```python
from build123d import *

# Parameters (mm, degrees)
BOSS_EXTRUDE1_DEPTH      = 10
BOSS_EXTRUDE2_DEPTH      = 1
BOSS_EXTRUDE2_DEPTH_BACK = 11
BOSS_EXTRUDE3_DEPTH      = 5
BOSS_EXTRUDE3_DEPTH_BACK = 5
BOSS_EXTRUDE4_DEPTH      = 5
BOSS_EXTRUDE4_DEPTH_BACK = 5
SKETCH19_R               = 1
CUT_EXTRUDE3_DEPTH       = 10
SKETCH24_R               = 1
CUT_EXTRUDE4_DEPTH       = 10
REVOLVE2_ANGLE           = 90
CUT_REVOLVE4_ANGLE       = 80


with BuildPart() as part:
    # Sketch1 → Boss-Extrude1 (new body)
    with BuildSketch(Plane.XY):
        with BuildLine():
            Line((186.280110435, 212.216863761), (189.127439812, 0))
            Line((189.127439812, 0), (0, 0))
            Line((0, 0), (0, 125.576698411))
            add(Edge.make_bspline(
                [(0, 125.576698411), (10.557001905, 132.837635912), (17.098165485, 150.751131911), (30.538510921, 175.76338894), (49.352217031, 203.04075133), (76.867896029, 207.296992896), (91.097956951, 209.776295723)],
                knots=[0, 0, 0, 0, 0.275246051, 0.426571591, 0.655828837, 1, 1, 1, 1], degree=3))
            add(Edge.make_bspline(
                [(91.097956951, 209.776295723), (122.565116695, 215.374757588), (154.60100966, 210.515513687), (186.280110435, 212.216863761)],
                knots=[0, 0, 0, 0, 1, 1, 1, 1], degree=3))
        make_face()
    extrude(amount=BOSS_EXTRUDE1_DEPTH)

    # Sketch3 → Boss-Extrude2 (add, two sides)
    with BuildSketch(Plane.XY.offset(10)) as boss_extrude2_sk:
        with BuildLine():
            Line((40.691917073, 127.565231362), (173.80372619, 127.565231362))
            Line((173.80372619, 127.565231362), (173.80372619, 199.679337801))
            add(Edge.make_bspline(
                [(40.691917073, 127.565231362), (46.771290341, 134.933306827), (53.369134393, 161.704453989), (78.457507643, 191.212262771), (124.31750344, 201.038762955), (152.264868916, 199.362802741), (173.80372619, 199.679337801)],
                knots=[0, 0, 0, 0, 0.16561761, 0.500501685, 0.611599227, 1, 1, 1, 1], degree=3))
        make_face()
    extrude(amount=BOSS_EXTRUDE2_DEPTH)
    extrude(boss_extrude2_sk.sketch, amount=-BOSS_EXTRUDE2_DEPTH_BACK)

    # Sketch17 → Boss-Extrude3 (add, two sides)
    with BuildSketch(Plane(origin=(0, 40, 0), x_dir=(-1, 0, 0), z_dir=(0, -1, 0))) as boss_extrude3_sk:
        with BuildLine():
            Line((-188.57501815, 0), (-189.57501815, 0))
            ThreePointArc((-189.57501815, 0), (-192.762810227, -4.99036016), (-189.57501815, -9.98072032))
            Line((-189.57501815, -9.98072032), (-188.57501815, -9.98072032))
            Line((-188.57501815, -9.98072032), (-188.57501815, 0))
        make_face()
    extrude(amount=BOSS_EXTRUDE3_DEPTH)
    extrude(boss_extrude3_sk.sketch, amount=-BOSS_EXTRUDE3_DEPTH_BACK)

    # Sketch18 → Boss-Extrude4 (add, two sides)
    with BuildSketch(Plane(origin=(0, 160, 0), x_dir=(-1, 0, 0), z_dir=(0, -1, 0))) as boss_extrude4_sk:
        with BuildLine():
            Line((-186.972854644, -10), (-187.472854644, -10))
            ThreePointArc((-187.472854644, -10), (-190.720096746, -5), (-187.472854644, 0))
            Line((-187.472854644, 0), (-186.972854644, 0))
            Line((-186.972854644, 0), (-186.972854644, -10))
        make_face()
    extrude(amount=BOSS_EXTRUDE4_DEPTH)
    extrude(boss_extrude4_sk.sketch, amount=-BOSS_EXTRUDE4_DEPTH_BACK)

    # Sketch19 → Cut-Extrude3 (cut)
    with BuildSketch(Plane.XZ.offset(-155)):
        with Locations((188.57501815, 5)):
            Circle(SKETCH19_R)
    extrude(amount=-CUT_EXTRUDE3_DEPTH, mode=Mode.SUBTRACT)

    # Sketch24 → Cut-Extrude4 (cut)
    with BuildSketch(Plane.XZ.offset(-35)):
        with Locations((190.94512502, 4.99518008)):
            Circle(SKETCH24_R)
    extrude(amount=-CUT_EXTRUDE4_DEPTH, mode=Mode.SUBTRACT)

    # Sketch30 → Revolve2 (revolve)
    with BuildSketch(Plane(origin=(0, 100, 0), x_dir=(1, 0, 0), z_dir=(0, 1, 0))):
        with BuildLine():
            Line((17.967687334, 0), (42.032312666, 0))
            ThreePointArc((42.032312666, 0), (30, 12.032312666), (17.967687334, 0))
        make_face()
    revolve(axis=Axis((17.967687334, 100, 0), (1, 0, 0)), revolution_arc=REVOLVE2_ANGLE)

    # Sketch31 → Cut-Revolve4 (revolve, cut)
    with BuildSketch(Plane.XZ.offset(-100)):
        with BuildLine():
            Line((20.003479707, 0), (39.804560833, 0))
            ThreePointArc((39.804560833, 0), (29.90402027, -9.900540563), (20.003479707, 0))
        make_face()
    revolve(axis=Axis((20.003479707, 100, 0), (1, 0, 0)), revolution_arc=CUT_REVOLVE4_ANGLE, mode=Mode.SUBTRACT)


solid = part.part
```
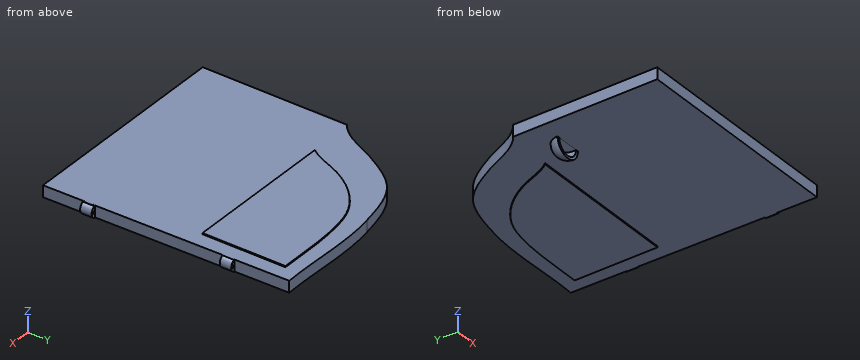
Part model, mm, in its own coordinate system. Round coordinates to 2 decimals unless told otherwise and drop trailing zeros. Write each loop counter-clockwise with the first axis right and the second up, starting at its lowest first coordinate (ties: lowest second). Pieces come first, ordered by that corner, then holes. Notation, with made-up numbers: M -6,11 L 27,11 A28 ccw 27,38 Z; hole C 73,70.5 d9. An arc over 180 degrees is marked long. Answer as CSV lines item,"result". Start each with the question number.
1) Drop flat-ended pins along their axis: pin 1 (0.8 mm diameter, centred on x = 113.5, z = -0.5, fed in from -Y); pin 2 (1 mm diameter, centred on x = 169.5, y = 143, fed in from -Z); pin 3 (12 mm diameter, centred on x = 21, y = 73, fed in from +Z). Give the stop position or say it passes through.
2) Band-saw the part on A-A (y = 104). List the corners of the cut face in (x, z) (3 decimals), then the cut area to 3 significant figures.
3) Drill centre lines: L1, parallel to Y at x = 128, z = 4.5; L2, parallel to Z at x = 125, y = 63.5; L3, parallel to X at y = 116, z = 0.75. Where is each one in solid material? Low to high.
Worked out:
1,pin 1,"y = 127.57"
1,pin 2,"z = -1"
1,pin 3,"z = 10"
2,outline,"M 0,0 L 18.652,0 A11.348 ccw 41.348,0 L 187.732,0 L 187.732,10 L 0,10 Z; hole M 20.875,-0.705 A9.057 ccw 38.933,-0.705 Z"
2,area,"1,960 mm²"
3,L1,"0 to 212.56"
3,L2,"0 to 10"
3,L3,"0 to 187.57"
